Here's the drawing with two shaded views (mm, measured from the low corner). I have some questions. Round coordinates to 2 decimals unless told otherwise and drop trailing zeros. Loops run counter-clockwise (first coordinate to the right, second up) from the corner with the lowest first, then second, coordinate; pieces in that order, holes last. Notation, with made-up numbers: (-35, 64.25) -> (22, 64.25) arc R15 ccw to (22, 89.25) -> close; hole circle Ø3 at (21.5, 42). An arc over 180 degrees is marked (long way). Write item = value, one per line.
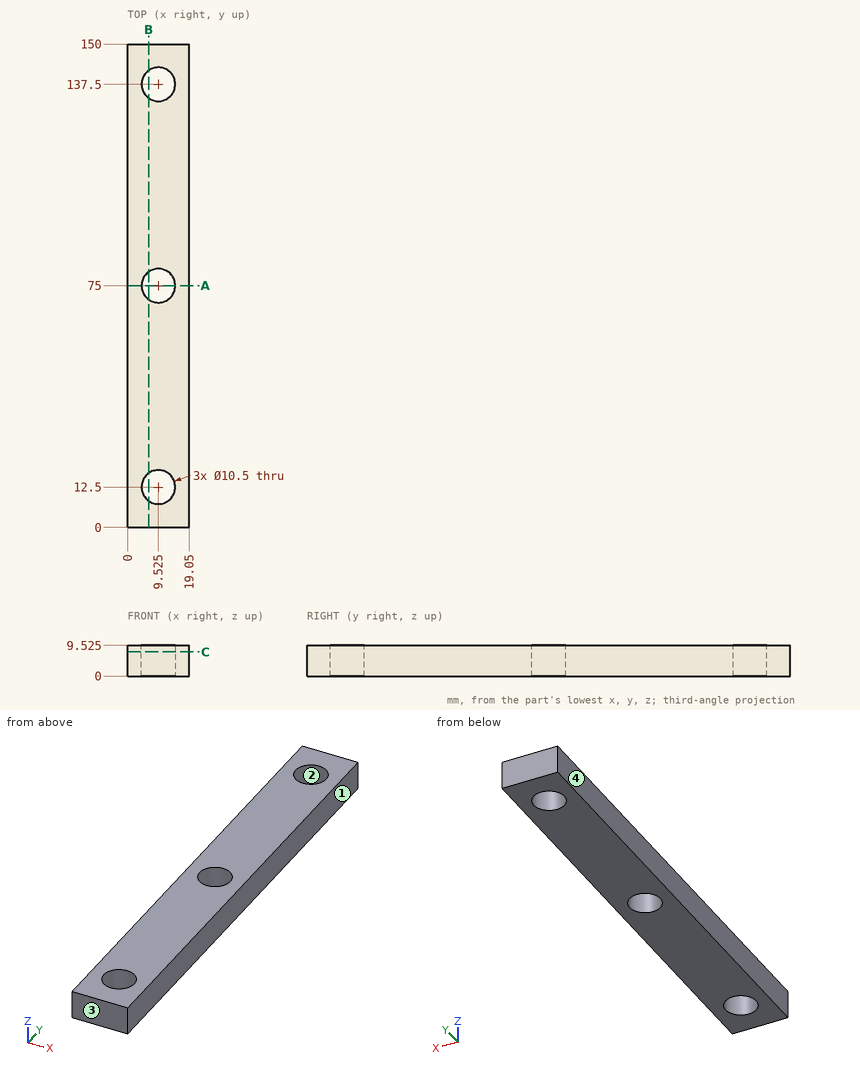
1. Suppose I cut it at A-A, the plane y = 75. List the corners of the cut face in (x, z) for me (3 decimals), and give its area (3 significant figures).
Entries:
outline = (0, 0) -> (4.275, 0) -> (4.275, 9.525) -> (0, 9.525) -> close; (14.775, 0) -> (19.05, 0) -> (19.05, 9.525) -> (14.775, 9.525) -> close
area = 81.4 mm²
2. Suppose I cut it at B-B, the plane x = 6.5. List the corners of the cut face in (y, z) for me (3 decimals).
Entries:
outline = (0, 0) -> (8.209, 0) -> (8.209, 9.525) -> (0, 9.525) -> close; (16.791, 0) -> (70.709, 0) -> (70.709, 9.525) -> (16.791, 9.525) -> close; (79.291, 0) -> (133.209, 0) -> (133.209, 9.525) -> (79.291, 9.525) -> close; (141.791, 0) -> (150, 0) -> (150, 9.525) -> (141.791, 9.525) -> close
3. I'm going to push a flat-ended pin straight in: pin 1 (1 mm diameter, centred on x = 5.5, y = 73.5, fed in from +Z). Where does the tip first touch, or does it pass through?
Entries:
pin_1 = through
4. I need wall thicknesses on line 1 (Y direction, x = 10, z = 9.25); line 2 (Y direction, x = 6, z = 5); line 3 (X direction, y = 137.5, z = 3.25) (3 decimals). Which ranges of each line are inside material? Lowest first, please. Write a range as [from, to].
Entries:
line_1 = [0, 7.27], [17.73, 69.77], [80.23, 132.27], [142.73, 150]
line_2 = [0, 8.61], [16.39, 71.11], [78.89, 133.61], [141.39, 150]
line_3 = [0, 4.275], [14.775, 19.05]
5. Suppose I cut it at C-C, the plane z = 7.5. List the corners of the cut face in (x, y) for me (3 decimals), and give its area (3 significant figures).
Entries:
outline = (0, 0) -> (19.05, 0) -> (19.05, 150) -> (0, 150) -> close; hole circle Ø10.5 at (9.525, 12.5); hole circle Ø10.5 at (9.525, 75); hole circle Ø10.5 at (9.525, 137.5)
area = 2,600 mm²
6. We'd pull the mould along X, two halves only. Please class the marked faces 1, 2, 3 and 4: released by +X, released by -X, zero draft, split by the parting line, or undercut.
Entries:
face_1 = released by +X
face_2 = undercut
face_3 = zero draft
face_4 = released by -X
